Model file for the job. Use its own axes, mm. Coordinates: 2 decimals unless noted, no trailing zeros. Write each loop counter-clockwise with the first axis right and the second up, starting at its lowest first coordinate (ties: lowest second). Pieces come first, ordered by that corner, then holes. Notation, with made-up numbers: M 8.5,79 L 43.5,79 A11 cw 43.5,99 Z; hole C -6.5,-26 d8. An arc over 180 degrees is marked long. One line per question, with ' | ' between items. Start each with the question number.
(1) Cut at A-A (x = -37.5). Write the cut outline in (y, z), plus the area to 3 significant figures.
(2) Cut at B-B (x = 22.5). Write the cut outline in (y, z).
(3) Cut at C-C (z = 0.8). Count the separate pieces of the cut face and the enclosed holes in it, plus the area to 3 significant figures.
(4) Wall check: probe 1 along Y at (x, z) = (-20.6, 2); probe 2 along Y at (x, z) = (-43, 0.5); probe 3 along X at (y, z) = (37.5, 1.9). Give the ranges that are in metal, low to high.
(5) Flat gauge pins, fed straight in: pin 1 Ø0.9 at (y, z) = (-63.5, 1) entering from +X; pin 2 Ø5 at (x, y) = (-20.6, -49.5) entering from +Z; pin 3 Ø1.5 at (y, z) = (70.5, 2) entering from +X; pin 4 Ø0.9 at (x, z) = (-73.5, 1) entering from +Y. Where does each tip first touch, or does it go through?
(6) Cut at D-D (y = -24.5). Write the cut outline in (x, z).
from build123d import *

# Parameters (mm, degrees)
CROQUIS1_W              = 10
CROQUIS1_H              = 3
CROQUIS1_W_2            = 28.1
CROQUIS1_H_2            = 15
CROQUIS1_R              = 1.5
CROQUIS1_W_3            = 29.3
SALIENTE_EXTRUIR3_DEPTH = 3


with BuildPart() as part:
    # Croquis1 → Saliente-Extruir3 (new body)
    with BuildSketch(Plane.XY):
        Polygon((-35, 72.5), (-45, 72.5), (-45, 69.5), (-55, 69.5), (-55, 72.5), (-65, 72.5), (-65, 69.5), (-75, 69.5), (-75, 62.5), (-72, 62.5), (-72, 52.5), (-75, 52.5), (-75, 42.5), (-72, 42.5), (-72, 32.5), (-75, 32.5), (-75, 22.5), (-72, 22.5), (-72, 12.5), (-75, 12.5), (-75, 2.5), (-72, 2.5), (-72, -7.5), (-75, -7.5), (-75, -17.5), (-72, -17.5), (-72, -27.5), (-75, -27.5), (-75, -37.5), (-72, -37.5), (-72, -47.5), (-75, -47.5), (-75, -50.25), (-65, -50.25), (-65, -53.25), (-75, -53.25), (-75, -57.5), (-72, -57.5), (-72, -69.5), (72, -69.5), (72, -57.5), (75, -57.5), (75, -53.25), (65, -53.25), (65, -50.25), (75, -50.25), (75, -47.5), (72, -47.5), (72, -37.5), (75, -37.5), (75, -27.5), (72, -27.5), (72, -17.5), (75, -17.5), (75, -7.5), (72, -7.5), (72, 2.5), (75, 2.5), (75, 12.5), (72, 12.5), (72, 22.5), (75, 22.5), (75, 32.5), (72, 32.5), (72, 42.5), (75, 42.5), (75, 52.5), (72, 52.5), (72, 62.5), (75, 62.5), (75, 69.5), (65, 69.5), (65, 72.5), (55, 72.5), (55, 69.5), (45, 69.5), (45, 72.5), (35, 72.5), (35, 69.5), (25, 69.5), (25, 72.5), (15, 72.5), (15, 69.5), (5, 69.5), (5, 72.5), (-5, 72.5), (-5, 69.5), (-15, 69.5), (-15, 72.5), (-25, 72.5), (-25, 69.5), (-35, 69.5), align=None)
        with Locations((60, 33)):
            Rectangle(CROQUIS1_W, CROQUIS1_H, mode=Mode.SUBTRACT)
        with Locations((-40.95, -58.25)):
            Rectangle(CROQUIS1_W_2, CROQUIS1_H_2, mode=Mode.SUBTRACT)
        with Locations((-20.6, -67)):
            Circle(CROQUIS1_R, mode=Mode.SUBTRACT)
        with Locations((-20.6, -49.5)):
            Circle(CROQUIS1_R, mode=Mode.SUBTRACT)
        with Locations((0.35, -58.25)):
            Rectangle(CROQUIS1_W_3, CROQUIS1_H_2, mode=Mode.SUBTRACT)
        with Locations((30, -51.75)):
            Rectangle(CROQUIS1_W, CROQUIS1_H, mode=Mode.SUBTRACT)
        with Locations((50, -51.75)):
            Rectangle(CROQUIS1_W, CROQUIS1_H, mode=Mode.SUBTRACT)
        with Locations((-60, 33)):
            Rectangle(CROQUIS1_W, CROQUIS1_H, mode=Mode.SUBTRACT)
        with Locations((-40, 33)):
            Rectangle(CROQUIS1_W, CROQUIS1_H, mode=Mode.SUBTRACT)
        Polygon((-25, 31.5), (-25, 34.5), (-17.5, 34.5), (-17.5, 49.5), (17.5, 49.5), (17.5, 34.5), (25, 34.5), (25, 31.5), (15, 31.5), (15, 34.5), (5, 34.5), (5, 31.5), (-5, 31.5), (-5, 34.5), (-15, 34.5), (-15, 31.5), align=None, mode=Mode.SUBTRACT)
        with Locations((40, 33)):
            Rectangle(CROQUIS1_W, CROQUIS1_H, mode=Mode.SUBTRACT)
    extrude(amount=SALIENTE_EXTRUIR3_DEPTH)


solid = part.part
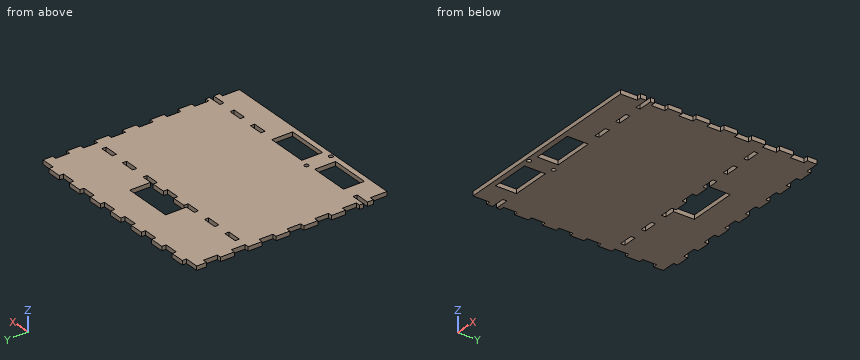
Filled in:
1) outline: M -69.5,0 L -65.75,0 L -65.75,3 L -69.5,3 Z; M -50.75,0 L 31.5,0 L 31.5,3 L -50.75,3 Z; M 34.5,0 L 72.5,0 L 72.5,3 L 34.5,3 Z | area: 372 mm²
2) outline: M -69.5,0 L 31.5,0 L 31.5,3 L -69.5,3 Z; M 34.5,0 L 72.5,0 L 72.5,3 L 34.5,3 Z
3) separate pieces: 1 | enclosed holes: 11 | area: 18,900 mm²
4) probe 1: -69.5 to -68.5, -65.5 to -51, -48 to 31.5, 34.5 to 72.5 | probe 2: -69.5 to -65.75, -50.75 to 31.5, 34.5 to 72.5 | probe 3: -72 to -17.5, 17.5 to 72
5) pin 1: x = 72 | pin 2: z = 3 | pin 3: x = 65 | pin 4: y = 69.5
6) outline: M -72,0 L 72,0 L 72,3 L -72,3 Z
